Print and shaded views of the part. All mm, measured from the part's lowest x, y and z. A direction names the side the tool comes from. Coordinates: 2 decimals unless noted, no trailing zeros. Order: outer loops, then holes, each group sorted by start corner. A loop starts at its lowest first (then second) coordinate and runs counter-clockwise, first axis right, second up.
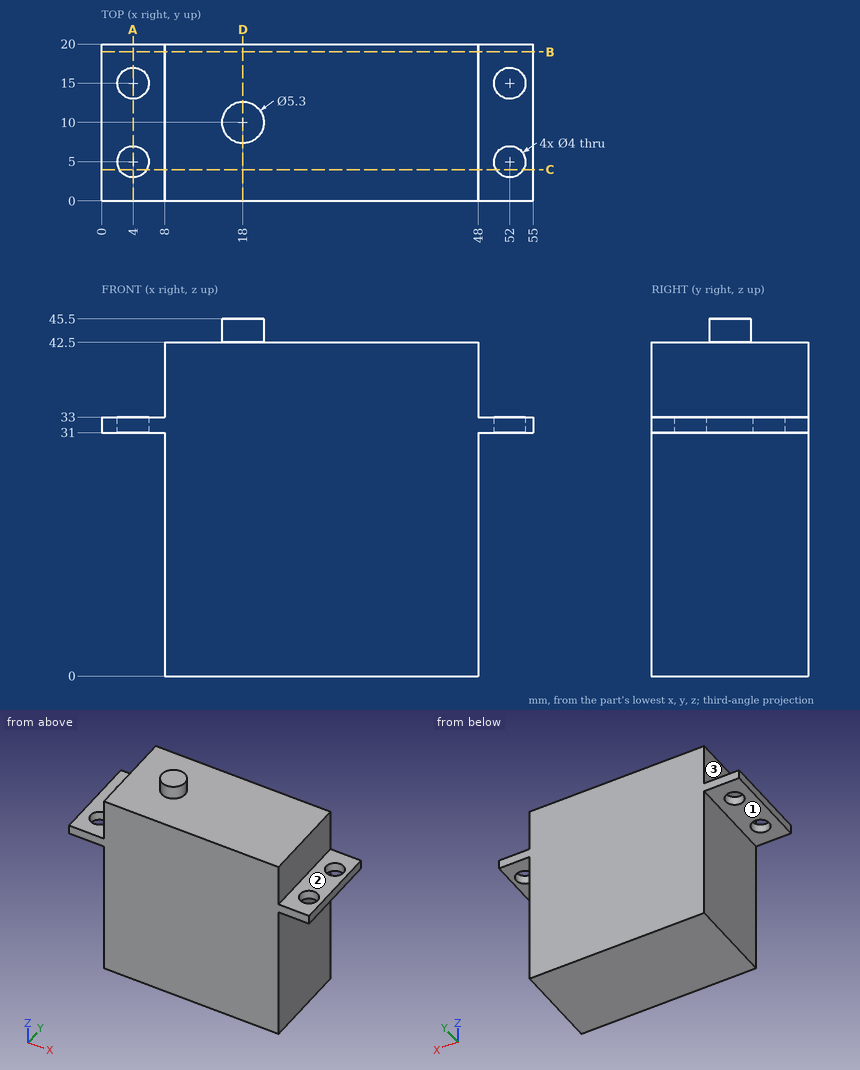
Q1. Cut at D-D, the plane x = 18. List the corners of the cut face in (y, z), plus the area to 3 significant figures.
Established:
outline: (0, 0) - (20, 0) - (20, 42.5) - (12.65, 42.5) - (12.65, 45.5) - (7.35, 45.5) - (7.35, 42.5) - (0, 42.5) - close
area: 866 mm2
Q2. Cut at A-A, the plane x = 4. List the corners of the cut face in (y, z).
Established:
outline: (0, 31) - (3, 31) - (3, 33) - (0, 33) - close; (7, 31) - (13, 31) - (13, 33) - (7, 33) - close; (17, 31) - (20, 31) - (20, 33) - (17, 33) - close
Q3. Cut at C-C, the plane y = 4. List the corners of the cut face in (x, z), plus the area to 3 significant figures.
Established:
outline: (0, 31) - (2.27, 31) - (2.27, 33) - (0, 33) - close; (5.73, 31) - (8, 31) - (8, 0) - (48, 0) - (48, 31) - (50.27, 31) - (50.27, 33) - (48, 33) - (48, 42.5) - (8, 42.5) - (8, 33) - (5.73, 33) - close; (53.73, 31) - (55, 31) - (55, 33) - (53.73, 33) - close
area: 1,720 mm2
Q4. Cut at B-B, the plane y = 19. List the corners of the cut face in (x, z).
Established:
outline: (0, 31) - (8, 31) - (8, 0) - (48, 0) - (48, 31) - (55, 31) - (55, 33) - (48, 33) - (48, 42.5) - (8, 42.5) - (8, 33) - (0, 33) - close
Q5. Which spindle directions (+Z, -Z, +X, -X, +Y, -Y) get a long thin tool onto all of the face, cutting with end or side? Do the marked faces 1, 2 and 3. Say none if no direction does.
Established:
face 1: -Z, -X, +Y, -Y
face 2: +Z, +X, +Y, -Y
face 3: +Z, -X, +Y, -Y
Q6. Drop flat-ended pins along their axis: P1, Ø4.5, axis at x = 4, y = 5, coming from the -Z side; P2, Ø7.5, axis at x = 51, y = 10, coming from the +Z side; P3, Ø6, axis at y = 7, z = 18, coming from the -X side. Give the stop position or say it passes through.
Established:
P1: stops at z = 31
P2: stops at z = 42.5
P3: stops at x = 8
Q7. Probe line 1 (Y direction, x = 4, z = 31.75); line 2 (Z direction, x = 7, y = 4.25); line 3 (Z direction, x = 37, y = 7.75). List the from-to ranges inside material, lowest first.
Established:
line 1: y = 0 to 3, 7 to 13, 17 to 20
line 2: z = 31 to 33
line 3: z = 0 to 42.5
